from build123d import *

# Parameters (mm, degrees)
BOX004_W         = 15
BOX004_H         = 26
BOX004_DEPTH     = 12
BOX005_W         = 9
BOX005_H         = 32
BOX005_DEPTH     = 8
FILLET004_R      = 2
PAD001_DEPTH     = 21
ARRAY001_Y_COUNT = 6
ARRAY001_Y_PITCH = 4
BOX003_W         = 25
BOX003_H         = 28
BOX003_DEPTH     = 18
FILLET003_R      = 2
FILLET005_R      = 2


with BuildPart() as cover_internal_cube:
    # Box004 → Box004 (new body)
    with BuildSketch(Plane(origin=(3, -3, -6), x_dir=(1, 0, 0), z_dir=(0, 0, 1))):
        with Locations((7.5, 13)):
            Rectangle(BOX004_W, BOX004_H)
    extrude(amount=BOX004_DEPTH)


with BuildPart() as middle_extract_cube_fillet001:
    # Box005 → Box005 (new body)
    with BuildSketch(Plane(origin=(6, -6, 10), x_dir=(1, 0, 0), z_dir=(0, 0, 1))):
        with Locations((4.5, 16)):
            Rectangle(BOX005_W, BOX005_H)
    extrude(amount=BOX005_DEPTH)

    # Fillet004
    fillet004_edges = [middle_extract_cube_fillet001.edges().sort_by_distance(p)[0] for p in [
        (6, 10, 10),
        (15, 10, 10),
    ]]
    fillet(fillet004_edges, radius=FILLET004_R)


with BuildPart() as extract_fusion001:
    # Sketch001 → Pad001 (new body)
    with BuildSketch(Plane.YZ):
        with BuildLine():
            Line((-0.7, 9), (-0.7, 2))
            Line((-0.7, 2), (0.7, 2))
            Line((0.7, 2), (0.7, 9))
            ThreePointArc((1, 12), (0.775187, 10.507481), (0.7, 9))
            Line((-1, 12), (1, 12))
            ThreePointArc((-0.7, 9), (-0.775187, 10.507481), (-1, 12))
        make_face()
    extrude(amount=PAD001_DEPTH)

    # Array001 Y: extract fusion001 ×6


with BuildPart() as extract_fusion001_1:
    add(extract_fusion001.part)
    with Locations(*[(0, i * ARRAY001_Y_PITCH, 0) for i in range(1, ARRAY001_Y_COUNT)]):
        add(extract_fusion001.part)

    # Fusion001: union cover internal cube, middle extract cube fillet001
    add(cover_internal_cube.part)
    add(middle_extract_cube_fillet001.part)


with BuildPart() as cover_glass_box_fillet:
    # Box003 → Box003 (new body)
    with BuildSketch(Plane(origin=(-2, -4, -6), x_dir=(1, 0, 0), z_dir=(0, 0, 1))):
        with Locations((12.5, 14)):
            Rectangle(BOX003_W, BOX003_H)
    extrude(amount=BOX003_DEPTH)

    # Fillet003
    fillet003_edges = [cover_glass_box_fillet.edges().sort_by_distance(p)[0] for p in [
        (-2, -4, 3),
        (-2, 24, 3),
        (23, -4, 3),
        (23, 24, 3),
    ]]
    fillet(fillet003_edges, radius=FILLET003_R)

    # Cut001: cut extract fusion001
    add(extract_fusion001_1.part, mode=Mode.SUBTRACT)

    # Fillet005
    fillet005_edges = [cover_glass_box_fillet.edges().sort_by_distance(p)[0] for p in [
        (6, 22.5, 12),
        (0, -4, 3),
        (3, -3, 0),
        (18, 14, 6),
    ]]
    fillet(fillet005_edges, radius=FILLET005_R)


solid = cover_glass_box_fillet.part
Design review of the part built by this model. Coordinates are the model's own, in mm. A direction names the side the tool comes from. Coordinates: 2 decimals unless noted, no trailing zeros. Loops run counter-clockwise (first coordinate to the right, second up) from the corner with the lowest first, then second, coordinate; pieces in that order, holes last.
Item 1: Wall thickness on L1, parallel to X at y = -1, z = 4.5; L2, parallel to Y at x = 7.5, z = 1.5; L3, parallel to X at y = 8.5, z = 4.5: over which ranges is each line inside the solid? List them lowest first.
Completed:
L1: x = -2 to 3, 18 to 23
L2: y = -4 to -3, 23 to 24
L3: x = -2 to 0, 21 to 23
Item 2: Add section D-D (y = 21.5). Write out the cut boundary in (x, z).
Completed:
outline: (-2, -6) - (3, -6) - (3, 6) - (18, 6) - (18, -6) - (23, -6) - (23, 12) - (15, 12) arc R2 cw to (13, 10) - (8, 10) arc R2 cw to (6.27, 11) arc R2 ccw to (4.54, 12) - (-2, 12) - close
Item 3: Add section B-B (x = 8.5). Give the number of separate pieces and of enclosed holes in the cut face, and give its area (3 significant figures).
Completed:
separate pieces: 7
enclosed holes: 0
area: 102 mm2
Item 4: Clearance check with flat-ended pins moving along their axes: pin 1 (5 mm diameter, centred on x = 16, y = 3.5, fed in from +Z); pin 2 (0.8 mm diameter, centred on x = 7, y = 14, fed in from -Z); pin 3 (0.7 mm diameter, centred on x = 1.5, y = 4, fed in from +Z); pin 4 (1 mm diameter, centred on x = 9, y = 11, fed in from +Z). State where each tip first meets the part, or that it passes through.
Completed:
pin 1: stops at z = 12
pin 2: stops at z = 6
pin 3: stops at z = 2
pin 4: stops at z = 10
Item 5: For faces 1 (the flat face through (0, 4, 7)), 2 (the cylindrical face through (14.43, 14.02, 10.6)), list the 3-axis set-ups (+Z, -Z, +X, -X, +Y, -Y) from which the entire face can be reached by the end or side of a thin tool; tool diameter is ignored.
Completed:
face 1: +Z
face 2: +Z, +Y, -Y
Item 6: Draft analysis for pull direction Y (two halves, no side actions). For faces 3 (the flat face through (21, 0, 7)), 4 (the cylindrical face through (22.43, 23.4, 3.13)), 5 (the cylindrical face through (6.57, 14.02, 10.6)), state which applies: pulls with the +Y half, pulls with the -Y half, needs draft (parallel to the pull), parting line crosses it, or undercut.
Completed:
face 3: undercut
face 4: pulls with the +Y half
face 5: needs draft
Item 7: Add section A-A (y = 12.25). Write out the cut boundary in (x, z), and give its area (3 significant figures).
Completed:
outline: (-2, -6) - (3, -6) - (3, 2) - (0, 2) - (0, 12) - (-2, 12) - close; (18, -6) - (23, -6) - (23, 12) - (21, 12) - (21, 2) - (18, 2) - close
area: 120 mm2
